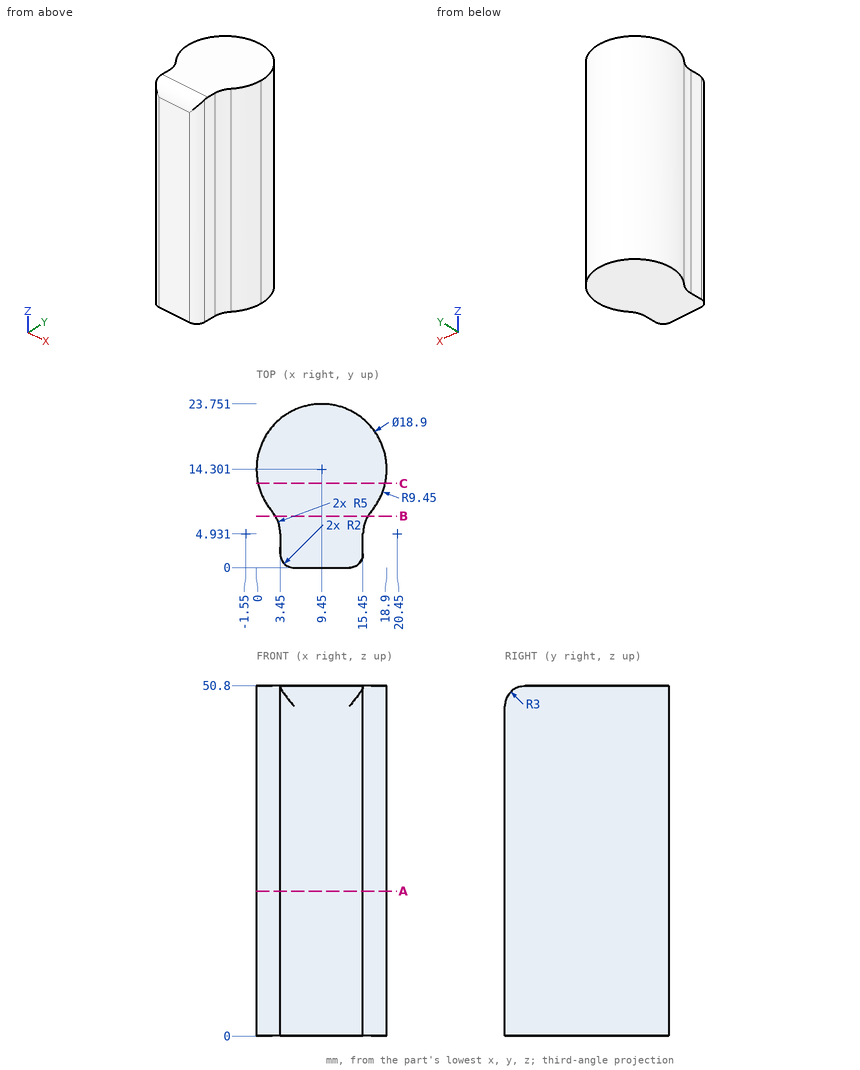
Source: three-view drawing plus pictorial views. Frame: mm from the lowest corner of the part. Give positions to 0.01 mm unless a question says otherwise; leave off trailing zeros. Write each loop counter-clockwise with the first axis right and the second up, starting at its lowest first coordinate (ties: lowest second). Pieces come first, ordered by that corner, then holes.
(1) Cut plane C-C, the plane y = 12.25. Return loops of the section in (x, z) (1 decimal), then the cut area to 3 significant figures.
(2) Ray query, line 1 (X direction, y = 4.25, z = 45); line 2 (X direction, y = 14.25, z = 4); line 3 (Y direction, x = 8.5, z = 39). Return the intervals inside material, ascending.
(3) Cut plane A-A, the plane z = 21. Return loops of the section in (x, y).
(4) Cut plane B-B, the plane y = 7.5. Return loops of the section in (x, z), then the cut area to 3 significant figures.
(5) First-contact query: P1, Ø1.5, axis at y = 11.5, z = 30, coming from the +X side (1 decimal); P2, Ø2.5, axis at y = 3, z = 19, coming from the -X side; P3, Ø4, axis at y = 11, z = 37, coming from the -X side; P4, Ø5, axis at y = 13, z = 36.5, coming from the +X side. Flat tips, straight axial feed; report the tip coordinate or a pass-through.
Values follow:
1. outline: (0.2, 0) - (18.7, 0) - (18.7, 50.8) - (0.2, 50.8) - close
1. area: 937 mm2
2. line 1: x = 3.45 to 15.45
2. line 2: x = 0 to 18.9
2. line 3: y = 0 to 23.7
3. outline: (2.26, 8.17) arc R5 cw to (3.45, 4.93) - (3.45, 2) arc R2 ccw to (5.45, 0) - (13.45, 0) arc R2 ccw to (15.45, 2) - (15.45, 4.93) arc R5 cw to (16.64, 8.17) arc R9.45 ccw (long way) to start
4. outline: (2.74, 0) - (16.16, 0) - (16.16, 50.8) - (2.74, 50.8) - close
4. area: 682 mm2
5. P1: stops at x = 18.7
5. P2: stops at x = 3.45
5. P3: stops at x = 0.09
5. P4: stops at x = 18.9
